Here's how the part is built. I have some questions about the finished solid (model axes, mm). Face numbers are marked on the shaded views. A direction names the side the tool comes from. Give positions to 0.01 mm unless a question says otherwise; leave off trailing zeros. Order: outer loops, then holes, each group sorted by start corner. A loop starts at its lowest first (then second) coordinate and runs counter-clockwise, first axis right, second up. Notation, with made-up numbers: (86, -2.75) -> (126, -2.75) arc R19 ccw to (126, 3.25) -> close; hole circle Ø8 at (31.25, 4.25). An arc over 180 degrees is marked (long way). Write each question's results on one line, items separated by ' | '. Start each with the question number.
Q1. I need wall thicknesses on line 1 along X through (y, z) = (5.9, 59.1); line 2 along X through (y, z) = (12.9, -59.6); line 3 along Z through (x, y) = (4, 5.75). Which ranges of each line are inside material? Lowest first, please. Write a range as [from, to].
Q2. Thinking about a two-plate mould opening in Z: for the marked faces 3, 4 and 5, which applies, pulls with the +Z half, pulls with the -Z half, needs draft (parallel to the pull), parting line crosses it, or undercut?
Q3. Imagine slicing it at D-D, the plane y = 26.5. Please give me the cut outline in (x, z), then the cut area to 3 significant figures.
Q4. Imagine slicing it at C-C, the plane x = -8. Please give me the cut outline in (y, z), then the cut area to 3 significant figures.
Q5. Imagine slicing it at B-B, the plane y = 5.9. Please give me the cut outline in (x, z), then the cut area to 3 significant figures.
Q6. I'm going to push flat-ended pins straight in: pin 1 (3 mm diameter, centred on x = -5, y = 12.9, fed in from +Z); pin 2 (2 mm diameter, centred on x = 1, y = 20.5, fed in from +Z); pin 3 (4 mm diameter, centred on x = 4, z = 56, fed in from +Y); pin 4 (3 mm diameter, centred on x = 0.5, z = 58, fed in from +Y). Where does each tip first touch, or does it pass through?
Q7. For the marked faces 1 and 2, which set-ups out of +Z, -Z, +X, -X, +Y, -Y let a thin tool reach every point of the face, with its end or its side?
```python
from build123d import *

# Parameters (mm, degrees)
BOSS_EXTRUDE1_DEPTH           = 8
M4_TAPPED_HOLE1_D             = 3.3
SKETCH8_W                     = 20
SKETCH8_H                     = 15
BOSS_EXTRUDE2_DEPTH           = 3
FILLET1_R                     = 1
M3_CLEARANCE_HOLE1_AT_2_COUNT = 2
M3_CLEARANCE_HOLE1_AT_2_PITCH = 13.03840481
FILLET1_OF_MIRROR1_R          = 1


with BuildPart() as part:
    # Sketch1 → Boss-Extrude1 (new body)
    with BuildSketch(Plane(origin=(0, 0, 0), x_dir=(0, 0, -1), z_dir=(1, 0, 0))):
        with BuildLine():
            Line((-60.995543931, 1.9), (-50.764456069, 1.9))
            ThreePointArc((-50.764456069, 1.9), (0, 50.8), (50.764456069, 1.9))
            Line((50.764456069, 1.9), (61.004456069, 1.9))
            Line((61.004456069, 1.9), (61.004456069, 16.9))
            Line((61.004456069, 16.9), (55.320249457, 16.9))
            ThreePointArc((55.320249457, 16.9), (54.442787227, 17.18342282), (53.896915423, 17.926586621))
            ThreePointArc((53.896915423, 17.926586621), (0, 56.8), (-53.896915423, 17.926586621))
            ThreePointArc((-53.896915423, 17.926586621), (-54.442787227, 17.18342282), (-55.320249457, 16.9))
            Line((-55.320249457, 16.9), (-60.995543931, 16.9))
            Line((-60.995543931, 16.9), (-60.995543931, 1.9))
        make_face()
    extrude(amount=BOSS_EXTRUDE1_DEPTH)

    # M4 Tapped Hole1 (through all)
    with Locations(Plane.XZ.offset(-1.9)):
        with Locations((4, -56.004456069), (4, 55.995543931)):
            Hole(M4_TAPPED_HOLE1_D / 2)

    # Sketch8 → Boss-Extrude2 (add)
    with BuildSketch(Plane.XY.offset(60.995543931)):
        with Locations((-10, 9.4)):
            Rectangle(SKETCH8_W, SKETCH8_H)
    boss_extrude2 = extrude(amount=-BOSS_EXTRUDE2_DEPTH)

    # Fillet1
    fillet1_edges = [part.edges().sort_by_distance(p)[0] for p in [
        (0, 9.4, 57.995543931),
    ]]
    fillet(fillet1_edges, radius=FILLET1_R)

    # Sketch9 → M3 Clearance Hole1 (revolve, cut)
    with BuildSketch(Plane(origin=(-5, 12.9, 57.995543931), x_dir=(0, 1, 0), z_dir=(1, 0, 0))):
        Polygon((0, 0), (0, 15.96137699), (1.6, 15), (1.6, 0), align=None)
    m3_clearance_hole1 = revolve(axis=Axis((-5, 12.9, 51.645543931), (0, 0, 1)), mode=Mode.SUBTRACT)

    # M3 Clearance Hole1 at 2: M3 Clearance Hole1 ×2
    with Locations(*[Vector(-0.8436614877321075, -0.5368754921931593, 0) * (i * M3_CLEARANCE_HOLE1_AT_2_PITCH) for i in range(1, M3_CLEARANCE_HOLE1_AT_2_COUNT)]):
        add(m3_clearance_hole1, mode=Mode.SUBTRACT)

    # Mirror1: Boss-Extrude2, M3 Clearance Hole1 across plane
    add(boss_extrude2.mirror(Plane(origin=(0, 0, -0.004456069), x_dir=(1, 0, 0), z_dir=(0, 0, -1))))
    add(m3_clearance_hole1.mirror(Plane(origin=(0, 0, -0.004456069), x_dir=(1, 0, 0), z_dir=(0, 0, -1))), mode=Mode.SUBTRACT)

    # Mirror1 copy 1 sketch → Mirror1 copy 1 (revolve, cut)
    with BuildSketch(Plane(origin=(-16, 5.9, -58.004456069), x_dir=(0, 1, 0), z_dir=(1, 0, 0))):
        Polygon((0, 0), (0, -15.96137699), (1.6, -15), (1.6, 0), align=None)
    revolve(axis=Axis((-16, 5.9, -51.654456069), (0, 0, 1)), mode=Mode.SUBTRACT)

    # Fillet1 of Mirror1
    fillet1_of_mirror1_edges = [part.edges().sort_by_distance(p)[0] for p in [
        (0, 9.4, -58.004456069),
    ]]
    fillet(fillet1_of_mirror1_edges, radius=FILLET1_OF_MIRROR1_R)


solid = part.part
```
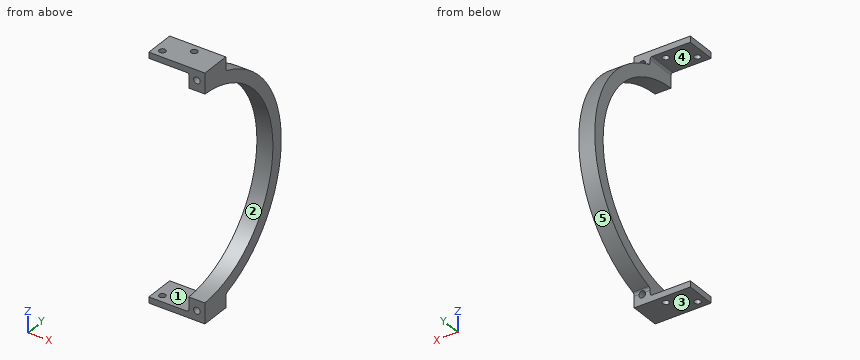
Geometry check:
1) line 1: [-20, -17.6], [-14.4, 8] | line 2: [-20, -6.6], [-3.4, 8] | line 3: [-61, -57.65], [-54.35, -50.47], [50.47, 54.35], [57.65, 61]
2) face 3: pulls with the -Z half | face 4: undercut | face 5: parting line crosses it
3) outline: (0, -50.24) -> (8, -50.24) -> (8, -43.34) -> (0, -43.34) -> close; (0, 43.34) -> (8, 43.34) -> (8, 50.24) -> (0, 50.24) -> close | area: 110 mm²
4) outline: (1.9, -61) -> (16.9, -61) -> (16.9, -58) -> (1.9, -58) -> close; (1.9, 58) -> (16.9, 58) -> (16.9, 61) -> (1.9, 61) -> close | area: 90.0 mm²
5) outline: (-20, -61) -> (-17.6, -61) -> (-17.6, -58) -> (-20, -58) -> close; (-20, 58) -> (-17.6, 58) -> (-17.6, 61) -> (-20, 61) -> close; (-14.4, -61) -> (8, -61) -> (8, -50.46) -> (0, -50.46) -> (0, -57) arc R1 cw to (-1, -58) -> (-14.4, -58) -> close; (-14.4, 58) -> (-1, 58) arc R1 cw to (0, 57) -> (0, 50.46) -> (8, 50.46) -> (8, 61) -> (-14.4, 61) -> close; hole circle Ø3.3 at (4, -56); hole circle Ø3.3 at (4, 56) | area: 253 mm²
6) pin 1: through | pin 2: z = 53.35 | pin 3: y = 17.69 | pin 4: y = 16.9
7) face 1: -X, +Y, -Y | face 2: +X, -X, -Y
